Autodesk Inventor part; units mm, degrees
ref_plane "Work Plane2" through (-40.9959, 0.8639, 22.2359) normal (0, 0, 1) x (1, 0, 0)
ref_plane "YZ Plane" through (0, 0, 0) normal (1, 0, 0) x (0, 1, 0)
ref_plane "XZ Plane" through (0, 0, 0) normal (0, 1, 0) x (-1, 0, 0)
ref_plane "Work Plane1" through (0, 0, 10) normal (0, 0, 1) x (1, 0, 0)
sketch "Sketch1" plane through (0, 0, 10) normal (0, 0, 1) x (1, 0, 0)
  line L0 (-4.0299, -0.3538) -> (-2.2322, 1.4439) construction
  arc A0 (-1.4439, 2.2322) -> (-2.2322, 1.4439) centre (-0.9299, 0.9299) ccw construction
  line L1 (-1.4439, 2.2322) -> (0.3538, 4.0299) construction
  line L2 (-37.8299, 42.8299) -> (-37.8299, 37.8299) construction
  line L3 (-37.8299, 37.8299) -> (-42.9208, 37.8299) construction
  line L4 (-37.8299, 42.2137) -> (-37.8299, 45.8299) construction
  line L5 (-37.8299, 45.8299) -> (-4.0299, 45.8299) construction
  line L6 (-4.0299, 45.8299) -> (-4.0299, 42.2137) construction
  line L7 (-4.0299, 4.0299) -> (0.3538, 4.0299)
  circle A1 centre (-20.9299, 20.9299) radius 17.5
  line L8 (-20.9299, 58.9723) -> (17.1124, 20.9299) construction
  line L9 (17.1124, 20.9299) -> (-20.9299, -17.1124) construction
  line L10 (-20.9299, -17.1124) -> (-58.9723, 20.9299) construction
  line L11 (-58.9723, 20.9299) -> (-20.9299, 58.9723) construction
  line L12 (-20.9299, 58.9723) -> (-20.9299, -17.1124) construction
  line L13 (17.1124, 20.9299) -> (-58.9723, 20.9299) construction
  line L14 (-20.9299, 58.9723) -> (32.8701, 58.9723) construction
  line L15 (-43.4299, 43.4299) -> (1.5701, 43.4299) construction
  line L16 (1.5701, 43.4299) -> (1.5701, -1.5701) construction
  line L17 (1.5701, -1.5701) -> (-43.4299, -1.5701) construction
  line L18 (-43.4299, -1.5701) -> (-43.4299, 43.4299) construction
  line L19 (-43.4299, 43.4299) -> (1.5701, -1.5701) construction
  line L20 (1.5701, 43.4299) -> (-43.4299, -1.5701) construction
  line L21 (-43.4299, 5.3876) -> (-43.4299, 36.4723)
  line L22 (-43.4299, 36.4723) -> (-36.4723, 43.4299)
  line L23 (-36.4723, 43.4299) -> (-5.3876, 43.4299)
  line L24 (-5.3876, 43.4299) -> (1.5701, 36.4723)
  line L25 (1.5701, 36.4723) -> (1.5701, 5.3876)
  line L26 (1.5701, 5.3876) -> (-5.3876, -1.5701)
  line L27 (-5.3876, -1.5701) -> (-36.4723, -1.5701)
  line L28 (-36.4723, -1.5701) -> (-43.4299, 5.3876)
  line L29 (-4.0299, 42.2137) -> (-37.8299, 42.2137)
  line L30 (-4.0299, -0.3538) -> (-4.0299, 4.0299)
  point P0 (-37.8299, 4.0299)
  point P1 (-20.9299, 20.9299)
  dimension "d18" = 53.8
  dimension "d19" = 45
  dimension "d20" = 53.8
  dimension "d21" = 45
  dimension "d22" = 45
extrude "Extrusion1" add sketch "Sketch1" along normal blind 10
sketch "Sketch2" plane through (0, 0, 20) normal (0, 0, 1) x (1, 0, 0)
  circle A0 centre (-35.9299, 35.9299) radius 3.0099 construction
  circle A1 centre (-5.93, 35.9299) radius 3.0099 construction
  circle A2 centre (-5.93, 5.93) radius 3.0099 construction
  circle A3 centre (-35.9299, 5.93) radius 3.0099 construction
  circle A4 centre (-35.9299, 35.9299) radius 2.925
  circle A5 centre (-5.93, 35.9299) radius 2.925
  circle A6 centre (-5.93, 5.93) radius 2.925
  circle A7 centre (-35.9299, 5.93) radius 2.925
  point P0 (0, 0)
  dimension "d1" = 5.85
  dimension "d31" = 5.85
  dimension "d32" = 5.85
  dimension "d33" = 5.85
ref_plane "Work Plane2" through (-40.9959, 0.8639, 22.2359) normal (0, 0, 1) x (1, 0, 0)
extrude "Extrusion2" add sketch "Sketch2" along normal blind 8
sketch "Sketch3" plane through (0, 0, 10) normal (0, 0, -1) x (-1, 0, 0)
  line L0 (37.8299, -0.4701) -> (37.8299, 4.0299) construction
  line L1 (4.0299, 4.0299) -> (4.0299, -0.4701) construction
  line L2 (37.8299, -0.4701) -> (37.8299, 1.1886) construction
  line L3 (4.0299, -3.9701) -> (4.0299, -0.3538) construction
  line L4 (45.8299, 4.0299) -> (42.2137, 4.0299) construction
  line L5 (-0.3538, 4.0299) -> (-3.9701, 4.0299) construction
  line L6 (-3.9701, 37.8299) -> (-0.3538, 37.8299) construction
  line L7 (4.0299, 42.2137) -> (4.0299, 45.8299) construction
  line L8 (37.8299, 45.8299) -> (37.8299, 42.2137) construction
  line L9 (42.2137, 37.8299) -> (45.8299, 37.8299) construction
  line L10 (40.4657, 37.7299) -> (45.8299, 37.7299)
  line L11 (45.8299, 37.7299) -> (45.8299, 4.1299)
  line L12 (45.8299, 4.1299) -> (40.4657, 4.1299)
  line L13 (40.4657, 4.1299) -> (40.4657, 37.7299)
  line L14 (37.7299, 2.4952) -> (4.1299, 2.4952)
  line L15 (4.1299, 2.4952) -> (4.1299, -3.9701)
  line L16 (4.1299, -3.9701) -> (37.7299, -3.9701)
  line L17 (37.7299, -3.9701) -> (37.7299, 2.4952)
  line L18 (1.8946, 4.1299) -> (-3.9701, 4.1299)
  line L19 (-3.9701, 4.1299) -> (-3.9701, 37.7299)
  line L20 (-3.9701, 37.7299) -> (1.8946, 37.7299)
  line L21 (1.8946, 37.7299) -> (1.8946, 4.1299)
  line L22 (4.1299, 40.7326) -> (37.7299, 40.7326)
  line L23 (37.7299, 40.7326) -> (37.7299, 45.8299)
  line L24 (37.7299, 45.8299) -> (4.1299, 45.8299)
  line L25 (4.1299, 45.8299) -> (4.1299, 40.7326)
  point P0 (0, 0)
  dimension "d23" = 0.1
  dimension "d24" = 0.1
  dimension "d25" = 0.1
  dimension "d26" = 0.1
  dimension "d27" = 0.1
extrude "Extrusion3" add sketch "Sketch3" against normal up to surface (10 mm away)
sketch "Sketch4" plane through (0, 0, 20) normal (0, 0, 1) x (1, 0, 0)
  line L0 (3.9701, 4.1299) -> (0.3124, 4.1299)
  line L1 (3.9701, 37.7299) -> (3.9701, 4.1299)
  line L2 (0.3124, 37.7299) -> (3.9701, 37.7299)
  line L3 (0.3124, 37.7299) -> (-4.1299, 42.1723)
  line L4 (-4.1299, 45.8299) -> (-4.1299, 42.1723)
  line L5 (-37.7299, 45.8299) -> (-4.1299, 45.8299)
  line L6 (-37.7299, 42.1723) -> (-37.7299, 45.8299)
  line L7 (-37.7299, 42.1723) -> (-42.1723, 37.7299)
  line L8 (-45.8299, 37.7299) -> (-42.1723, 37.7299)
  line L9 (-45.8299, 4.1299) -> (-45.8299, 37.7299)
  line L10 (-42.1723, 4.1299) -> (-45.8299, 4.1299)
  line L11 (-42.1723, 4.1299) -> (-37.7299, -0.3124)
  line L12 (-37.7299, -3.9701) -> (-37.7299, -0.3124)
  line L13 (-4.1299, -3.9701) -> (-37.7299, -3.9701)
  line L14 (-4.1299, -0.3124) -> (-4.1299, -3.9701)
  line L15 (-4.1299, -0.3124) -> (0.3124, 4.1299)
  circle A0 centre (-20.9299, 20.9299) radius 17.5
  circle A1 centre (-35.9299, 5.93) radius 2.925
  circle A2 centre (-5.93, 35.9299) radius 2.925
  circle A3 centre (-35.9299, 35.9299) radius 2.925
  circle A4 centre (-5.93, 5.93) radius 2.925
  line L16 (-3.9799, 45.9799) -> (-3.9799, 42.2344)
  line L17 (-3.9799, 42.2344) -> (0.3745, 37.8799)
  line L18 (0.3745, 37.8799) -> (4.1201, 37.8799)
  line L19 (4.1201, 37.8799) -> (4.1201, 3.9799)
  line L20 (4.1201, 3.9799) -> (0.3745, 3.9799)
  line L21 (0.3745, 3.9799) -> (-3.9799, -0.3745)
  line L22 (-3.9799, -0.3745) -> (-3.9799, -4.1201)
  line L23 (-3.9799, -4.1201) -> (-37.8799, -4.1201)
  line L24 (-37.8799, -4.1201) -> (-37.8799, -0.3745)
  line L25 (-37.8799, -0.3745) -> (-42.2344, 3.9799)
  line L26 (-42.2344, 3.9799) -> (-45.9799, 3.9799)
  line L27 (-45.9799, 3.9799) -> (-45.9799, 37.8799)
  line L28 (-45.9799, 37.8799) -> (-42.2344, 37.8799)
  line L29 (-42.2344, 37.8799) -> (-37.8799, 42.2344)
  line L30 (-37.8799, 42.2344) -> (-37.8799, 45.9799)
  line L31 (-37.8799, 45.9799) -> (-3.9799, 45.9799)
  point P0 (0, 0)
  dimension "d34" = 0.15
extrude "Extrusion4" add sketch "Sketch4" against normal up to surface (10 mm away) contours L16 L17 L18 L19 L20 L21 L22 L23 L24 L25 L26 L27 L28 L29 L30 L31
ref_plane "Arbeitsebene3" through (-37.8799, 20.9299, 20) normal (0, -1, 0) x (1, 0, 0)
ref_plane "Arbeitsebene4" through (-20.9299, 3.9799, 20) normal (1, 0, 0) x (0, 0, -1)
equation "\"d31\" = d1"
equation "\"d32\" = d1"
equation "\"d33\" = d1"
properties part number "20_Cube_Insert_Thorlabs_Pins"
Here's how the part is built. I have some questions about the finished solid (model axes, mm). A direction names the side the tool comes from. Give positions to 0.01 mm unless a question says otherwise; leave off trailing zeros. Order: outer loops, then holes, each group sorted by start corner. A loop starts at its lowest first (then second) coordinate and runs counter-clockwise, first axis right, second up. Notation, with made-up numbers: (40, -12) -> (45, -12) arc R30 ccw to (45, 24) -> close; hole circle Ø2 at (76.5, 47.25). An arc over 180 degrees is marked (long way). Use a Markdown table: item, result. Add a question column.
Item 1: Imagine slicing it at D-D on x = -5.93. Please give me the cut outline in (y, z) (3 decimals).
Item 2: Imagine slicing it at A-A on x = -14. Please give me the cut outline in (y, z), plus the area to 3 significant figures.
Item 3: Will these pins go through, and if not, where does the flat tip stop? pin 1 (5 mm diameter, centred on y = 37, z = 25, fed in from -X); pin 2 (1.9 mm diameter, centred on x = -44, z = 12.5, fed in from -Y); pin 3 (4 mm diameter, centred on y = -2.5, z = 12.5, fed in from -X).
Item 4: I need wall thicknesses on line 1 (Y direction, x = -42.5, z = 11.5); line 2 (X direction, y = 34, z = 12.25); line 3 (X direction, y = 8.5, z = 23.75). Which ranges of each line are inside material? Lowest first, please.
Item 5: If we mould it in two halves opening along Y, with no side actions, what happens to faces 5 (the face through (-44, 37.88, 15)), 6 (the face through (-45.98, 21, 15)), 7 (the face through (-38.852, 5.801, 23.944)), 8 (the face through (-21, -4.12, 15))? For each: pulls with the +Y half, pulls with the -Y half, needs draft (parallel to the pull), parting line crosses it, or undercut.
Item 6: For faces 1 (the face through (2, 37.88, 15)), 2 (the face through (-37.88, -2, 15)), 3 (the face through (2, 3.98, 15)), 4 (the face through (-38.086, 33.953, 23.944)), which set-ups out of +Z, -Z, +X, -X, +Y, -Y let a thin tool reach every point of the face, with its end or its side?
Item 7: Imagine slicing it at C-C on z = 12.5. Please give me the cut outline in (x, y), plus the area to 3 significant figures.
Item 8: Imagine slicing it at B-B on y = 5.93. Please give me the cut outline in (x, z) (3 decimals), plus the area to 3 significant figures.
Data:
| question | item | result |
|---|---|---|
| 1 | outline | (-4.12, 10) -> (11.916, 10) -> (11.916, 20) -> (8.855, 20) -> (8.855, 28) -> (3.005, 28) -> (3.005, 20) -> (-4.12, 20) -> close; (29.944, 10) -> (45.98, 10) -> (45.98, 20) -> (38.855, 20) -> (38.855, 28) -> (33.005, 28) -> (33.005, 20) -> (29.944, 20) -> close |
| 2 | outline | (-4.12, 10) -> (4.86, 10) -> (4.86, 20) -> (-4.12, 20) -> close; (37, 10) -> (45.98, 10) -> (45.98, 20) -> (37, 20) -> close |
| 2 | area | 180 mm² |
| 3 | pin 1 | stops at x = -38.85 |
| 3 | pin 2 | stops at y = 3.98 |
| 3 | pin 3 | stops at x = -37.88 |
| 4 | line 1 | y = 3.98 to 37.88 |
| 4 | line 2 | x = -45.98 to -32.57, -9.29 to 4.12 |
| 4 | line 3 | x = -37.33 to -34.53, -7.33 to -4.53 |
| 5 | face 5 | pulls with the +Y half |
| 5 | face 6 | needs draft |
| 5 | face 7 | undercut |
| 5 | face 8 | pulls with the -Y half |
| 6 | face 1 | +Z, -Z, +X, +Y |
| 6 | face 2 | +Z, -Z, -X, -Y |
| 6 | face 3 | +Z, -Z, +X, -Y |
| 6 | face 4 | +Z |
| 7 | outline | (-45.98, 3.98) -> (-42.23, 3.98) -> (-37.88, -0.37) -> (-37.88, -4.12) -> (-3.98, -4.12) -> (-3.98, -0.37) -> (0.37, 3.98) -> (4.12, 3.98) -> (4.12, 37.88) -> (0.37, 37.88) -> (-3.98, 42.23) -> (-3.98, 45.98) -> (-37.88, 45.98) -> (-37.88, 42.23) -> (-42.23, 37.88) -> (-45.98, 37.88) -> close; hole circle Ø35 at (-20.93, 20.93) |
| 7 | area | 1,320 mm² |
| 8 | outline | (-45.98, 10) -> (-29.944, 10) -> (-29.944, 20) -> (-33.005, 20) -> (-33.005, 28) -> (-38.855, 28) -> (-38.855, 20) -> (-45.98, 20) -> close; (-11.916, 10) -> (4.12, 10) -> (4.12, 20) -> (-3.005, 20) -> (-3.005, 28) -> (-8.855, 28) -> (-8.855, 20) -> (-11.916, 20) -> close |
| 8 | area | 414 mm² |
